from build123d import *

# Parameters (mm, degrees)
F2_R      = 139.7
F3_DEPTH  = 19.05
F4_SIZE   = 1.5875
F5_R      = 120.65
F6_DEPTH  = 19.051
F7_R      = 0.79375
F8_DEPTH  = 19.051
F9_R      = 4.7625
F9_R_2    = 0.79375
F10_DEPTH = 15.875


# Not quite as in the source:
# - a variable given as a bare number and used for a length is read in inches; the dataset says mm whatever the document's units were


with BuildPart() as f3:
    # F2 (on Top) → F3 (new body)
    with BuildSketch(Plane.XY):
        Circle(F2_R)
    extrude(amount=F3_DEPTH)

    # F4
    f4_edges = [f3.edges().sort_by_distance(p)[0] for p in [
        (-139.7, 0, 19.05),
        (-139.7, 0, 0),
    ]]
    chamfer(f4_edges, length=F4_SIZE)

    # F5 (on face) → F6 (cut, through all)
    with BuildSketch(Plane(origin=(0, 0, 0), x_dir=(1, 0, 0), z_dir=(0, 0, -1))):
        Circle(F5_R)
    extrude(amount=-F6_DEPTH, mode=Mode.SUBTRACT)

    # F7 (on face) → F8 (cut, through all)
    with BuildSketch(Plane.XY.offset(19.05)):
        with Locations((0, 130.175)):
            Circle(F7_R)
        with Locations((130.175, 0)):
            Circle(F7_R)
        with Locations((0, -130.175)):
            Circle(F7_R)
        with Locations((-130.175, 0)):
            Circle(F7_R)
    extrude(amount=-F8_DEPTH, mode=Mode.SUBTRACT)

    # F9 (on face) → F10 (cut)
    with BuildSketch(Plane.XY.offset(19.05)):
        with Locations((0, 130.175)):
            Circle(F9_R)
        with Locations((0, 130.175)):
            Circle(F9_R_2, mode=Mode.SUBTRACT)
        with Locations((130.175, 0)):
            Circle(F9_R)
        with Locations((130.175, 0)):
            Circle(F9_R_2, mode=Mode.SUBTRACT)
        with Locations((-130.175, 0)):
            Circle(F9_R)
        with Locations((-130.175, 0)):
            Circle(F9_R_2, mode=Mode.SUBTRACT)
        with Locations((0, -130.175)):
            Circle(F9_R)
        with Locations((0, -130.175)):
            Circle(F9_R_2, mode=Mode.SUBTRACT)
    extrude(amount=-F10_DEPTH, mode=Mode.SUBTRACT)


solid = f3.part
Can you work these out from the model? Positions are in its coordinate system, mm. A direction names the side the tool comes from. Coordinates: 2 decimals unless noted, no trailing zeros. Answer as CSV lines item,"result".
(1) Suppose I cut it at A-A on z = 6.75. Count the separate pieces of the cut face and the enclosed holes in it, plus the area to 3 significant figures.
Geometry check:
separate pieces,"1"
enclosed holes,"5"
area,"15,300 mm^2"
(2) I'm going to push flat-ended pins straight in: pin 1 (3 mm diameter, centred on x = -73.5, z = 4.5, fed in from -Y); pin 2 (12.5 mm diameter, centred on x = 0, y = 130.175, fed in from -Z); pin 3 (1.5 mm diameter, centred on y = -91.5, z = 8, fed in from +X); pin 4 (3 mm diameter, centred on y = -111.5, z = 11.5, fed in from -X). Where does each tip first touch, or does it pass through?
Geometry check:
pin 1,"y = -119.72"
pin 2,"z = 0"
pin 3,"x = 106.21"
pin 4,"x = -86.12"
(3) If we mould it in two halves opening along Y, with no side actions, what happens to faces 1 (the flat face through (122, 1, 19.05)), 2 (the cylindrical face through (-110.86, -85.01, 9.41)), 3 (the flat face through (131.2, 0.1, 3.175)), 4 (the flat face through (-0.1, -131.2, 3.175))? For each: released by +Y, released by -Y, zero draft, split by the parting line, or undercut.
Geometry check:
face 1,"zero draft"
face 2,"split by the parting line"
face 3,"undercut"
face 4,"undercut"
(4) On a 3-axis mill with a long thin cutter (end or side, diameter ignored), from which of +Z, -Z, +X, -X, +Y, -Y can I reach the whole of each face in a straight line? I mean faces 5 (the flat face through (1, 130, 3.175)), 6 (the cylindrical face through (-120.533, -5.305, 9.392)). Say none if no direction works.
Geometry check:
face 5,"+Z"
face 6,"+Z, -Z"
(5) Please list where these lines run through material, in increasing order: L1, parallel to Y at x = -47, z = 3.25; L2, parallel to Y at x = 9, z = 15; L3, parallel to X at y = 27.5, z = 6.
Geometry check:
L1,"-131.56 to -111.12, 111.12 to 131.56"
L2,"-139.41 to -120.31, 120.31 to 139.41"
L3,"-136.97 to -117.47, 117.47 to 136.97"
